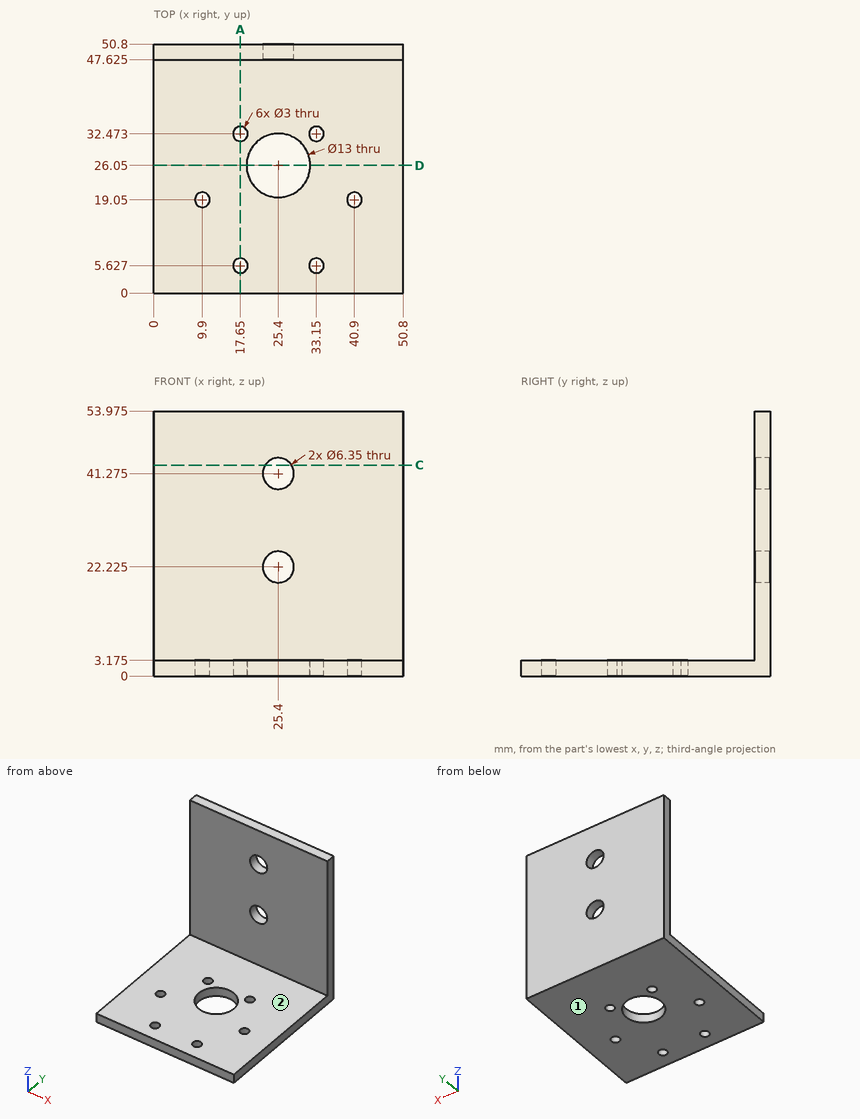
Answer from the drawing. Dimensions are ordinates in mm from the lowest x, y and z of the part. A direction names the side the tool comes from. Give positions to 0.01 mm unless a question says otherwise; leave off trailing zeros. Loops run counter-clockwise (first coordinate to the right, second up) from the corner with the lowest first, then second, coordinate; pieces in that order, holes last. Notation, with made-up numbers: (55, 68) -> (91, 68) arc R32 cw to (91, 103) -> close; hole circle Ø6 at (5, -18.5). An arc over 180 degrees is marked (long way). Use a Markdown table: item, result.
Q1. Find the intervals of material crossed by line 1 along Y through (x, z) = (33, 1) (1 decimal); line 2 along Z through (x, y) = (24, 13) (1 decimal); line 3 along Y through (x, z) = (31.5, 6.5) (1 decimal), in increasing order.
Solved:
| item | result |
|---|---|
| line 1 | y = 0 to 4.1, 7.1 to 31, 34 to 50.8 |
| line 2 | z = 0 to 3.2 |
| line 3 | y = 47.6 to 50.8 |
Q2. A tool of negligible diameter and unlimited length cuts with its end or side. For the marked faces 1 and 2, from which of +Z, -Z, +X, -X, +Y, -Y can it reach the whole face along a straight path? Write none if from no direction.
Solved:
| item | result |
|---|---|
| face 1 | -Z, +X, -X, +Y, -Y |
| face 2 | +Z, +X, -X, -Y |
Q3. Section C-C, the plane z = 43 is taken. Determine the outline of the cut face in (x, y) (1 decimal).
Solved:
| item | result |
|---|---|
| outline | (0, 47.6) -> (22.7, 47.6) -> (22.7, 50.8) -> (0, 50.8) -> close; (28.1, 47.6) -> (50.8, 47.6) -> (50.8, 50.8) -> (28.1, 50.8) -> close |
Q4. Each of these flat-tipped pins is pushed along its axis until it touches: pin 1 (8 mm diameter, centred on x = 7.5, y = 16.5, fed in from +Z) (3 decimals); pin 2 (1.5 mm diameter, centred on x = 21.5, z = 27, fed in from -Y) (3 decimals); pin 3 (1.8 mm diameter, centred on x = 17.65, y = 32.47, fed in from -Z). Where does it stop, or does it pass through?
Solved:
| item | result |
|---|---|
| pin 1 | stops at z = 3.175 |
| pin 2 | stops at y = 47.625 |
| pin 3 | passes through |
Q5. Section A-A, the plane x = 17.65 is taken. Determine the outline of the cut face in (y, z) (1 decimal).
Solved:
| item | result |
|---|---|
| outline | (0, 0) -> (4.1, 0) -> (4.1, 3.2) -> (0, 3.2) -> close; (7.1, 0) -> (31, 0) -> (31, 3.2) -> (7.1, 3.2) -> close; (34, 0) -> (50.8, 0) -> (50.8, 54) -> (47.6, 54) -> (47.6, 3.2) -> (34, 3.2) -> close |
Q6. Section D-D, the plane y = 26.05 is taken. Determine the outline of the cut face in (x, z) (1 decimal).
Solved:
| item | result |
|---|---|
| outline | (0, 0) -> (18.9, 0) -> (18.9, 3.2) -> (0, 3.2) -> close; (31.9, 0) -> (50.8, 0) -> (50.8, 3.2) -> (31.9, 3.2) -> close |
